from build123d import *

# Parameters (mm, degrees)
BOSS_EXTRUDE1_DEPTH = 12.7
SKETCH2_R           = 1.5875
CUT_EXTRUDE1_DEPTH  = 19.05
CUT_EXTRUDE2_DEPTH  = 3.175
FILLET2_R           = 2.54
FILLET3_R           = 1.27
SKETCH3_R           = 1.086795662
BOSS_EXTRUDE2_DEPTH = 2.54
FILLET4_R           = 0.762
SKETCH4_R           = 0.491571792
CUT_EXTRUDE3_DEPTH  = 2.54


with BuildPart() as part:
    # Sketch1 → Boss-Extrude1 (new body)
    with BuildSketch(Plane(origin=(0, 0, 0), x_dir=(0, 0, -1), z_dir=(1, 0, 0))):
        with BuildLine():
            Line((-4.7625, 0), (-4.7625, 27.9908))
            ThreePointArc((-4.7625, 27.9908), (0, 32.7533), (4.7625, 27.9908))
            Line((4.7625, 27.9908), (4.7625, 0))
            ThreePointArc((4.7625, 0), (0, -4.7625), (-4.7625, 0))
        make_face()
    extrude(amount=BOSS_EXTRUDE1_DEPTH)

    # Sketch2 → Cut-Extrude1 (cut)
    with BuildSketch(Plane(origin=(12.7, 0, 0), x_dir=(0, 0, -1), z_dir=(1, 0, 0))):
        Circle(SKETCH2_R)
        with Locations((0, 27.9908)):
            Circle(SKETCH2_R)
    extrude(amount=-CUT_EXTRUDE1_DEPTH, mode=Mode.SUBTRACT)

    # 3DSketch1 → Cut-Extrude2 (cut, symmetric)
    with BuildSketch(Plane(origin=(6.35, 27.9908, -4.7625), x_dir=(0, -0.9466889316456175, 0.322149137356721), z_dir=(1, 0, 0))):
        with BuildLine():
            Line((0, 0), (4.508606037, 1.534235267))
            Line((4.508606037, 1.534235267), (7.57707657, -7.482976807))
            Line((7.57707657, -7.482976807), (3.068470533, -9.017212074))
            ThreePointArc((3.068470533, -9.017212074), (-2.97437077, -6.042841304), (0, 0))
        make_face()
        with BuildLine():
            Line((29.567051081, 0), (25.058445044, -1.534235267))
            Line((25.058445044, -1.534235267), (21.989974511, 7.482976807))
            Line((21.989974511, 7.482976807), (26.498580548, 9.017212074))
            ThreePointArc((26.498580548, 9.017212074), (32.541421852, 6.042841304), (29.567051081, 0))
        make_face()
    extrude(amount=CUT_EXTRUDE2_DEPTH, both=True, mode=Mode.SUBTRACT)

    # Fillet2
    fillet2_edges = [part.edges().sort_by_distance(p)[0] for p in [
        (6.35, 23.2283, -4.7625),
        (6.35, 4.7625, -4.7625),
        (6.35, 4.7625, 4.7625),
        (6.35, 23.2283, 4.7625),
    ]]
    fillet(fillet2_edges, radius=FILLET2_R)

    # Fillet3
    fillet3_edges = [part.edges().sort_by_distance(p)[0] for p in [
        (12.7, 32.7533, 0),
        (12.7, 13.9954, 4.7625),
        (9.525, 24.33955, 4.7625),
        (9.525, 24.33955, -4.7625),
        (3.175, 24.33955, -4.7625),
        (3.175, 24.33955, 4.7625),
        (12.7, -4.7625, 0),
        (0, 13.9954, 4.7625),
        (0, 32.7533, 0),
        (9.525, 3.65125, -4.7625),
        (9.525, 3.65125, 4.7625),
        (0, 13.9954, -4.7625),
        (3.175, 3.65125, 4.7625),
        (3.175, 3.65125, -4.7625),
        (0, -4.7625, 0),
        (12.7, 13.9954, -4.7625),
    ]]
    fillet(fillet3_edges, radius=FILLET3_R)

    # Sketch3 → Boss-Extrude2 (add)
    with BuildSketch(Plane.ZY):
        with Locations((-2.225739377, 2.096022994)):
            Circle(SKETCH3_R)
    extrude(amount=BOSS_EXTRUDE2_DEPTH)

    # Fillet4
    fillet4_edges = [part.edges().sort_by_distance(p)[0] for p in [
        (-2.54, 2.096022994, -3.312535039),
    ]]
    fillet(fillet4_edges, radius=FILLET4_R)

    # Sketch4 → Cut-Extrude3 (cut)
    with BuildSketch(Plane(origin=(0, 3.476983319, -2.007437255), x_dir=(-1, 0, 0), z_dir=(0, 0.8660254037844399, -0.4999999999999979))):
        with Locations(Location((0.856605906, -0.806785971, 0), (0, 0, 90))):
            Circle(SKETCH4_R)
    extrude(amount=-CUT_EXTRUDE3_DEPTH, mode=Mode.SUBTRACT)


solid = part.part
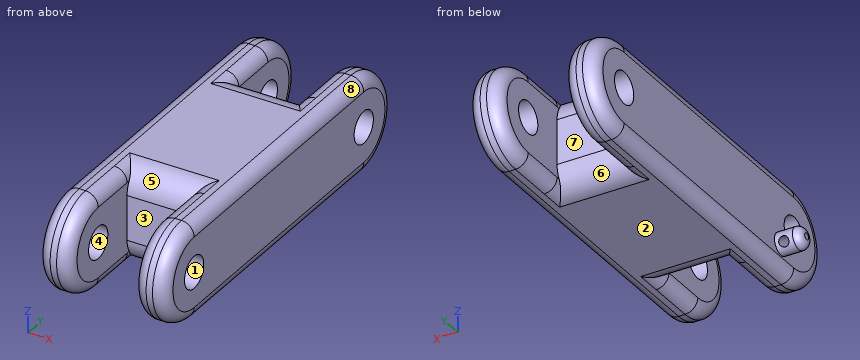
Read the model definition and answer for the solid it produces. Units are mm, in the model's axes. Face numbers are marked on the shaded views. A direction names the side the tool comes from. Coordinates: 2 decimals unless noted, no trailing zeros. Loops run counter-clockwise (first coordinate to the right, second up) from the corner with the lowest first, then second, coordinate; pieces in that order, holes last.
Q1. The part is cut by section B-B on x = 7.25. Write down the section's boundary in (y, z), and give its area (3 significant figures).
Q2. The part is cut by section C-C on y = 16. Write down the section's boundary in (x, z), and give its area (3 significant figures).
Q3. Which of the six approach directions +Z, -Z, +X, -X, +Y, -Y give full straight-line access (tool end or side, diameter ignored) to the marked faces 4, 5, 6, 7 and 8?
Q4. Each of these flat-tipped pins is pushed along its axis until it touches: pin 1 Ø2 at (x, z) = (5.5, 0) entering from +Y; pin 2 Ø1 at (x, z) = (10.5, -2.5) entering from +Y; pin 3 Ø5.5 at (y, z) = (13.5, -1.5) entering from -X. Where does it stop, or does it pass through?
Q5. Consider probe 1 along Y at (x, z) = (1.75, 0); probe 2 along X at (y, z) = (-2, 1.5) (3 decimals); probe 3 along Y at (x, z) = (11.9, 0). Determine where each line is inside the solid, lowest interval first.
Q6. The part is cut by section A-A on y = 24.5. Write down the section's boundary in (x, z) (1 decimal).
Q7. The part is cut by section D-D on z = 0. Give the number of separate pieces and of enclosed holes in the cut face, and give its area (3 significant figures).
Q8. The mould has two halves that part along Y. Classify the marked faces 1, 2 and 3: +Y half, -Y half, draft (parallel to the pull), parting line (faces both ways), or undercut.
Results below:
1. outline: (4.76, -2.22) arc R2.54 ccw to (7.3, -4.76) - (20.69, -4.76) arc R2.54 ccw to (23.23, -2.22) - (23.23, 2.22) arc R2.54 ccw to (20.69, 4.76) - (7.3, 4.76) arc R2.54 ccw to (4.76, 2.22) - close
1. area: 170 mm2
2. outline: (0, -3.49) arc R1.27 ccw to (1.27, -4.76) - (11.43, -4.76) arc R1.27 ccw to (12.7, -3.49) - (12.7, 3.49) arc R1.27 ccw to (11.43, 4.76) - (1.27, 4.76) arc R1.27 ccw to (0, 3.49) - close
2. area: 120 mm2
3. face 4: +X, -X
3. face 5: +Z, -Y
3. face 6: -Z, +Y
3. face 7: +Z, -Z, +Y
3. face 8: +Z, +X, +Y, -Y
4. pin 1: stops at y = 23.23
4. pin 2: stops at y = 32.29
4. pin 3: stops at x = 0
5. probe 1: y = -4.76 to -1.59, 1.59 to 26.4, 29.58 to 32.75
5. probe 2: x = 0 to 3.175, 9.525 to 12.7
5. probe 3: y = -4.67 to -1.59, 1.59 to 26.4, 29.58 to 32.66
6. outline: (0, -3.5) arc R1.3 ccw to (1.3, -4.8) - (1.9, -4.8) arc R1.3 ccw to (3.2, -3.5) - (3.2, 3.5) arc R1.3 ccw to (1.9, 4.8) - (1.3, 4.8) arc R1.3 ccw to (0, 3.5) - close; (9.5, -3.5) arc R1.3 ccw to (10.8, -4.8) - (11.4, -4.8) arc R1.3 ccw to (12.7, -3.5) - (12.7, 3.5) arc R1.3 ccw to (11.4, 4.8) - (10.8, 4.8) arc R1.3 ccw to (9.5, 3.5) - close
7. separate pieces: 5
7. enclosed holes: 0
7. area: 312 mm2
8. face 1: undercut
8. face 2: draft
8. face 3: -Y half
